from build123d import *

# Parameters (mm, degrees)
SKETCH1_W           = 57.18
SKETCH1_H           = 50.8
BOSS_EXTRUDE1_DEPTH = 18
SKETCH2_R           = 11
CUT_EXTRUDE1_DEPTH  = 58
FILLET2_R           = 18
FILLET3_R           = 18


with BuildPart() as part:
    # Sketch1 → Boss-Extrude1 (new body)
    with BuildSketch(Plane(origin=(0, 0, 0), x_dir=(1, 0, 0), z_dir=(0, 1, 0))):
        with Locations((-6.481243802, 7.033465199)):
            Rectangle(SKETCH1_W, SKETCH1_H)
    extrude(amount=BOSS_EXTRUDE1_DEPTH)

    # Sketch2 → Cut-Extrude1 (cut)
    with BuildSketch(Plane.ZY.offset(35.071243802)):
        with Locations((-7.033465199, 0)):
            Circle(SKETCH2_R)
    extrude(amount=-CUT_EXTRUDE1_DEPTH, mode=Mode.SUBTRACT)

    # Fillet2
    fillet2_edges = [part.edges().sort_by_distance(p)[0] for p in [
        (-6.481243802, 18, 18.366534801),
    ]]
    fillet(fillet2_edges, radius=FILLET2_R - 0.0001)  # a hair under: the kernel refuses the full size

    # Fillet3
    fillet3_edges = [part.edges().sort_by_distance(p)[0] for p in [
        (-6.481243802, 18, -32.433465199),
    ]]
    fillet(fillet3_edges, radius=FILLET3_R - 0.0001)  # a hair under: the kernel refuses the full size


solid = part.part
Could you check a few things on this model? Use its own coordinates, in mm. Coordinates: 2 decimals unless noted, no trailing zeros. Write each loop counter-clockwise with the first axis right and the second up, starting at its lowest first coordinate (ties: lowest second). Pieces come first, ordered by that corner, then holes. Notation, with made-up numbers: (81.5, 15.25) - (140.5, 15.25) arc R14 ccw to (140.5, 30.25) - close; hole circle Ø4 at (72.25, 86). An arc over 180 degrees is marked (long way). Write item = value, one per line.
1) Suppose I cut it at D-D on z = 8. Please give me the cut outline in (x, y), plus the area to 3 significant figures.
Result set:
outline = (-35.07, 0) - (22.11, 0) - (22.11, 16.3) - (-35.07, 16.3) - close
area = 932 mm2
2) Suppose I cut it at C-C on y = 2.25. Please give me the cut outline in (x, z), plus the area to 3 significant figures.
Result set:
outline = (-35.07, -32.29) - (22.11, -32.29) - (22.11, -17.8) - (-35.07, -17.8) - close; (-35.07, 3.73) - (22.11, 3.73) - (22.11, 18.23) - (-35.07, 18.23) - close
area = 1,660 mm2
3) Suppose I cut it at A-A on y = 7.75. Please give me the cut outline in (x, z), plus the area to 3 significant figures.
Result set:
outline = (-35.07, -30.68) - (22.11, -30.68) - (22.11, -14.84) - (-35.07, -14.84) - close; (-35.07, 0.77) - (22.11, 0.77) - (22.11, 16.61) - (-35.07, 16.61) - close
area = 1,810 mm2
4) We'd pull the mould along Z, two halves only. Please class faces 1 (the cylindrical face through (-6.08, 12.87, -27.02)), 2 (the cylindrical face through (-7, 11, -7)), 3 (the flat face through (-7, 18, -7)), 4 (the cylindrical face through (-6.08, 12.87, 12.95)): +Z half, -Z half, draft (parallel to the pull), parting line (faces both ways), or undercut.
Result set:
face_1 = -Z half
face_2 = undercut
face_3 = draft
face_4 = +Z half
5) Will these pins go through, and if not, where does the flat tip stop? pin 1 Ø3 at (x, z) = (8.5, -23.5) entering from +Y; pin 2 Ø5 at (x, y) = (7, 7.5) entering from -Z; pin 3 Ø6 at (x, y) = (-8.5, 9.5) entering from -Z.
Result set:
pin_1 = 16.33
pin_2 = -31.73
pin_3 = -31.22
6) Please list where these lines run through material, in increasing order: line 1 (Z direction, x = -17, y = 9); line 2 (Z direction, x = -16.5, y = 5); line 3 (Y direction, x = -25.5, z = 1.5). Write a range as [from, to].
Result set:
line_1 = [-30.02, -13.36], [-0.71, 15.96]
line_2 = [-31.73, -16.83], [2.76, 17.66]
line_3 = [6.94, 17.96]
